Verification items for the finished model (mm, model axes). Face numbers are marked on the shaded views. A direction names the side the tool comes from. Round coordinates to 2 decimals unless told otherwise and drop trailing zeros. Order: outer loops, then holes, each group sorted by start corner. A loop starts at its lowest first (then second) coordinate and runs counter-clockwise, first axis right, second up. Notation, with made-up numbers: M 42,27 L 97,27 A23 cw 97,35 Z; hole C 67.25,75.5 d8. An arc over 180 degrees is marked long. Use CSV: the item, a comma, the result in double quotes. Start each with the question number.
Q1. Set-up check for the marked faces 1 and 2: record each of +Z, -Z, +X, -X, +Y, -Y from which the full face is reachable in a straight line by a thin tool's end or side.
Q2. Gauge pin test, flat ends, axial feed: pin 1 Ø1.9 at (x, z) = (0, 10.5) entering from +Y; pin 2 Ø13 at (x, y) = (-6.5, 2.5) entering from +Z; pin 3 Ø2.5 at (x, z) = (-3, 11) entering from +Y. Record the tip position at first contact, or that the pin passes through.
Q3. Sectioned sample at C-C (y = 5). Enter the section's corners in (x, z).
Q4. Mould release check, pull along Y, two halves, no side actions. Record for the marked faces 3, 4, 5 and 6: +Y half, -Y half, draft (parallel to the pull), parting line (faces both ways), or undercut.
Q5. Scan lines: line 1 (X direction, y = -18.2, z = 10.5); line 2 (X direction, y = 6, z = 4.5); line 3 (Z direction, x = 3, y = 9). Record each from-to range of solid material in increasing order.
Q6. Sectioned sample at D-D (z = 4). Enter the section's corners in (x, y), and give its area (3 significant figures).
Q7. Sectioned sample at B-B (z = 11.25). Enter the section's corners in (x, y).
Q8. Sectioned sample at A-A (x = 3.25). Enter the section's corners in (y, z), and give its area (3 significant figures).
```python
from build123d import *

# Parameters (mm, degrees)
SKETCH_1_R          = 7.5
SKETCH_1_R_2        = 1.25
EXTRUDE_1_DEPTH     = 5.5
SKETCH_2_W          = 26
SKETCH_2_H          = 4
EXTRUDE_2_DEPTH     = 9
SKETCH_3_R          = 1.6
CUT_EXTRUDE_1_DEPTH = 12
FILLET_1_R          = 2


with BuildPart() as part:
    # 草图1 → 凸台-拉伸1 (new body)
    with BuildSketch(Plane.XY):
        with BuildLine():
            Line((-13, 0), (-13, -20))
            Line((-13, -20), (13, -20))
            Line((13, -20), (13, 0))
            ThreePointArc((13, 0), (0, 13), (-13, 0))
        make_face()
        Circle(SKETCH_1_R, mode=Mode.SUBTRACT)
        with Locations((-7.071067812, 7.071067812)):
            Circle(SKETCH_1_R_2, mode=Mode.SUBTRACT)
        with Locations((7.071067812, 7.071067812)):
            Circle(SKETCH_1_R_2, mode=Mode.SUBTRACT)
        with Locations((7.071067812, -7.071067812)):
            Circle(SKETCH_1_R_2, mode=Mode.SUBTRACT)
        with Locations((-7.071067812, -7.071067812)):
            Circle(SKETCH_1_R_2, mode=Mode.SUBTRACT)
    extrude(amount=EXTRUDE_1_DEPTH)

    # 草图2 → 凸台-拉伸2 (add)
    with BuildSketch(Plane.XY.offset(5.5)):
        with Locations((0, -18)):
            Rectangle(SKETCH_2_W, SKETCH_2_H)
    extrude(amount=EXTRUDE_2_DEPTH)

    # 草图3 → 切除-拉伸1 (cut)
    with BuildSketch(Plane(origin=(0, -16, 0), x_dir=(1, 0, 0), z_dir=(0, 1, 0))):
        with Locations(Location((-10, -10.5, 0), (0, 0, 270))):
            Circle(SKETCH_3_R)
        with Locations(Location((0, -10.5, 0), (0, 0, 270))):
            Circle(SKETCH_3_R)
        with Locations(Location((10, -10.5, 0), (0, 0, 270))):
            Circle(SKETCH_3_R)
    extrude(amount=-CUT_EXTRUDE_1_DEPTH, mode=Mode.SUBTRACT)

    # 圆角1
    fillet_1_edges = [part.edges().sort_by_distance(p)[0] for p in [
        (-13, -18, 14.5),
        (13, -18, 14.5),
    ]]
    fillet(fillet_1_edges, radius=FILLET_1_R)


solid = part.part
```
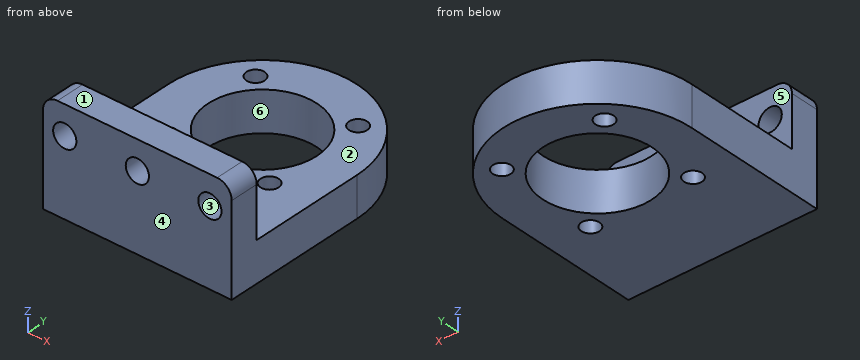
Verdict:
1,face 1,"+Z, +X, -X, +Y, -Y"
1,face 2,"+Z, +X, -X, +Y"
2,pin 1,"passes through"
2,pin 2,"stops at z = 5.5"
2,pin 3,"stops at y = -16"
3,outline,"M -12,0 L -5.59,0 L -5.59,5.5 L -12,5.5 Z; M 5.59,0 L 12,0 L 12,5.5 L 5.59,5.5 Z"
4,face 3,"draft"
4,face 4,"-Y half"
4,face 5,"+Y half"
4,face 6,"undercut"
5,line 1,"x = -13 to -11.6, -8.4 to -1.6, 1.6 to 8.4, 11.6 to 13"
5,line 2,"x = -11.53 to -7.72, -6.43 to -4.5, 4.5 to 6.43, 7.72 to 11.53"
5,line 3,"z = 0 to 5.5"
6,outline,"M -13,-20 L 13,-20 L 13,0 A13 ccw -13,0 Z; hole C -7.07,-7.07 d2.5; hole C -7.07,7.07 d2.5; hole C 0,0 d15; hole C 7.07,-7.07 d2.5; hole C 7.07,7.07 d2.5"
6,area,"589 mm²"
7,outline,"M -13,-20 L -11.41,-20 L -11.41,-16 L -13,-16 Z; M -8.59,-20 L -1.41,-20 L -1.41,-16 L -8.59,-16 Z; M 1.41,-20 L 8.59,-20 L 8.59,-16 L 1.41,-16 Z; M 11.41,-20 L 13,-20 L 13,-16 L 11.41,-16 Z"
8,outline,"M -20,0 L -6.76,0 L -6.76,5.5 L -16,5.5 L -16,14.5 L -20,14.5 Z; M 6.76,0 L 12.59,0 L 12.59,5.5 L 6.76,5.5 Z"
8,area,"141 mm²"
